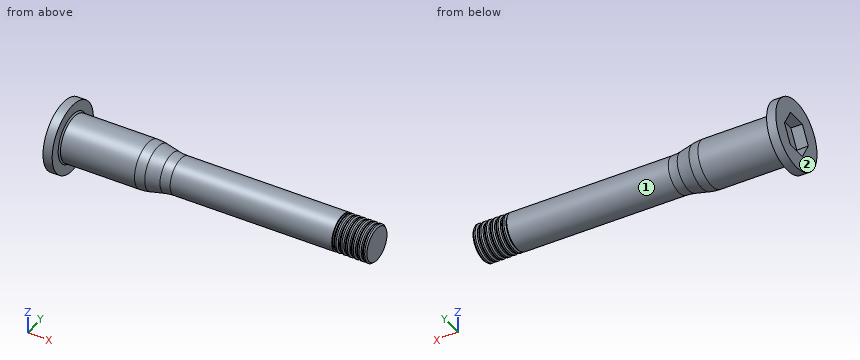
from build123d import *

# Parameters (mm, degrees)
LPATTERN1_COUNT    = 6
LPATTERN1_PITCH    = 3.175
CUT_EXTRUDE1_DEPTH = 6.35
FILLET1_R          = 25.4
CHAMFER1_SIZE      = 0.79375


with BuildPart() as part:
    # Sketch2 → Revolve1 (revolve)
    with BuildSketch(Plane.XY, mode=Mode.PRIVATE) as revolve1_sk:
        Polygon((-5.08, 0), (168.275, 0), (168.275, 10), (57.15, 10), (44.45, 12.7127), (0, 12.7127), (0, 19.05), (-5.08, 19.05), align=None)
    revolve(revolve1_sk.sketch.rotate(Axis((-8.585810146, 0, 0), (1, 0, 0)), 90), axis=Axis((-8.585810146, 0, 0), (1, 0, 0)))

    # Sketch3 → Cut-Revolve1 (revolve, cut)
    with BuildSketch(Plane.XY, mode=Mode.PRIVATE) as cut_revolve1_sk:
        Polygon((168.275, 9.2634), (167.438897849, 10.0254), (166.6875, 10.0254), (165.851397849, 9.2634), (165.1, 9.2634), (165.1, 10.5334), (168.275, 10.5334), align=None)
    cut_revolve1 = revolve(cut_revolve1_sk.sketch.rotate(Axis((-8.585810146, 0, 0), (1, 0, 0)), 90), axis=Axis((-8.585810146, 0, 0), (1, 0, 0)), mode=Mode.SUBTRACT)

    # LPattern1: Cut-Revolve1 ×6
    with Locations(*[(-i * LPATTERN1_PITCH, 0, 0) for i in range(1, LPATTERN1_COUNT)]):
        add(cut_revolve1, mode=Mode.SUBTRACT)

    # Sketch4 → Cut-Extrude1 (cut)
    with BuildSketch(Plane.ZY.offset(5.08)):
        Polygon((0, 10.998522628), (-9.525, 5.499261314), (-9.525, -5.499261314), (0, -10.998522628), (9.525, -5.499261314), (9.525, 5.499261314), align=None)
    extrude(amount=-CUT_EXTRUDE1_DEPTH, mode=Mode.SUBTRACT)

    # Fillet1
    fillet1_edges = [part.edges().sort_by_distance(p)[0] for p in [
        (57.15, 0, -10),
        (44.45, 0, -12.7127),
    ]]
    fillet(fillet1_edges, radius=FILLET1_R)

    # Chamfer1
    chamfer1_edges = [part.edges().sort_by_distance(p)[0] for p in [
        (0, 0, -12.7127),
    ]]
    chamfer(chamfer1_edges, length=CHAMFER1_SIZE)


solid = part.part
Here's how the part is built. I have some questions about the finished solid (model axes, mm). Face numbers are marked on the shaded views. A direction names the side the tool comes from. Coordinates: 2 decimals unless noted, no trailing zeros. Order: outer loops, then holes, each group sorted by start corner. A loop starts at its lowest first (then second) coordinate and runs counter-clockwise, first axis right, second up. Notation, with made-up numbers: (10.25, -32.5) - (27.25, -32.5) arc R30 cw to (27.25, -0.5) - close; hole circle Ø11 at (-31, -37). An arc over 180 degrees is marked (long way). Use CSV: the item, a comma, the result in double quotes. Start each with the question number.
1. I'm going to push flat-ended pins straight in: pin 1 (2 mm diameter, centred on y = -5.5, z = -13, fed in from +X); pin 2 (12 mm diameter, centred on x = 130.5, y = 9.5, fed in from -Z); pin 3 (4 mm diameter, centred on x = 82, z = -8.5, fed in from +Y). Where does each tip first touch, or does it pass through?
2. Suppose I cut it at C-C on x = 14.5. List the corners of the cut face in (y, z) for me, then the cut area to 3 significant figures.
3. Suppose I cut it at B-B on z = -15. List the corners of the cut face in (x, y) for me, then the cut area to 3 significant figures.
4. Please list where these lines run through material, in increasing order: line 1 (X direction, y = -16, z = -1.5); line 2 (X direction, y = 9, z = -1) (3 decimals); line 3 (Y direction, x = 132, z = 0). Write a range as from..to.
5. For the marked faces 1 and 2, which set-ups out of +Z, -Z, +X, -X, +Y, -Y let a thin tool reach every point of the face, with its end or its side?
6. Suppose I cut it at A-A on x = 136. List the corners of the cut face in (y, z) for me.
Output:
1,pin 1,"stops at x = 0.39"
1,pin 2,"stops at z = -9.37"
1,pin 3,"stops at y = 7.6"
2,outline,"circle Ø25.43 at (0, 0)"
2,area,"508 mm2"
3,outline,"(-5.08, -11.74) - (0, -11.74) - (0, 11.74) - (-5.08, 11.74) - close"
3,area,"119 mm2"
4,line 1,"x = -5.08..0"
4,line 2,"x = 1.27..168.275"
4,line 3,"y = -10..10"
5,face 1,"+X"
5,face 2,"+Z, -Z, -X, +Y, -Y"
6,outline,"circle Ø20 at (0, 0)"
